Here's the drawing with two shaded views (mm, measured from the low corner). I have some questions. A direction names the side the tool comes from. Give positions to 0.01 mm unless a question says otherwise; leave off trailing zeros. Loops run counter-clockwise (first coordinate to the right, second up) from the corner with the lowest first, then second, coordinate; pieces in that order, holes last. Notation, with made-up numbers: (-27, 25.5) - (-16, 25.5) arc R34 ccw to (-16, 61.5) - close; hole circle Ø5 at (-36, -11). An arc over 180 degrees is marked (long way). Use one line per item in the form item = value.
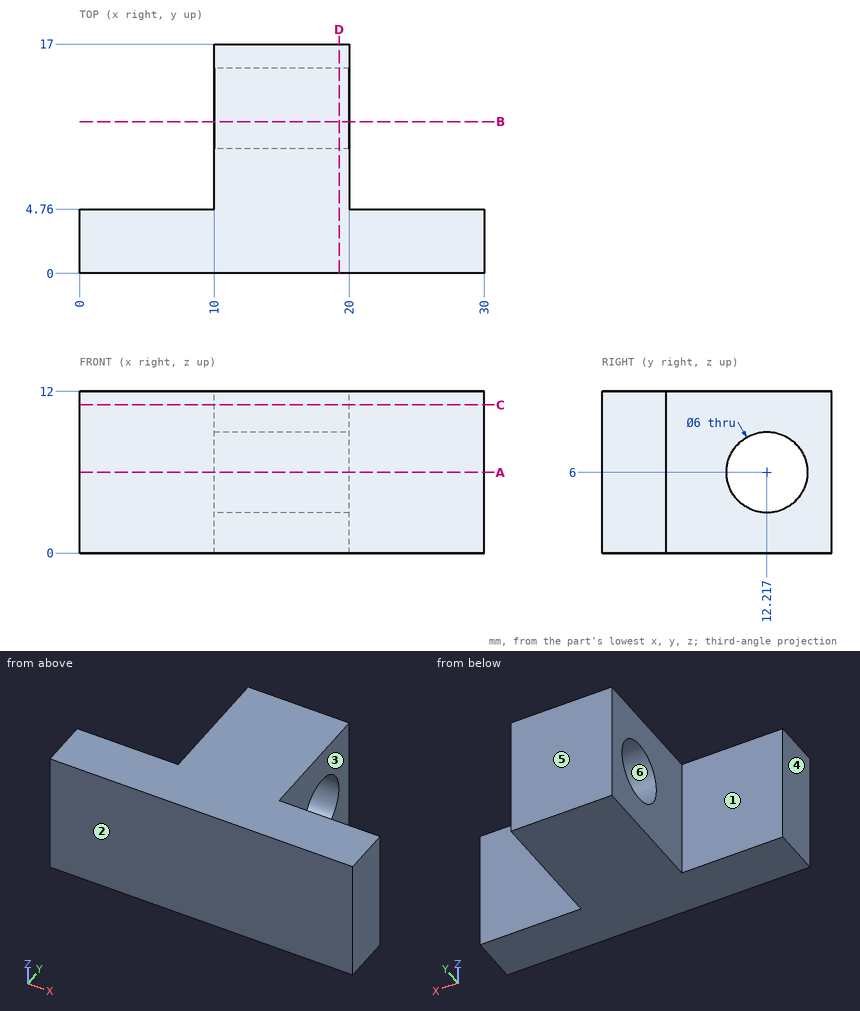
(1) If we section it at C-C (z = 11): List the corners of the cut face in (x, y) for me.
Geometry says:
outline = (0, 0) - (30, 0) - (30, 4.76) - (20, 4.76) - (20, 17) - (10, 17) - (10, 4.76) - (0, 4.76) - close
(2) If we section it at D-D (x = 19.25): List the corners of the cut face in (y, z) for me.
Geometry says:
outline = (0, 0) - (17, 0) - (17, 12) - (0, 12) - close; hole circle Ø6 at (12.22, 6)
(3) If we section it at B-B (y = 11.25): List the corners of the cut face in (x, z) for me, plus the area to 3 significant figures.
Geometry says:
outline = (10, 0) - (20, 0) - (20, 3.16) - (10, 3.16) - close; (10, 8.84) - (20, 8.84) - (20, 12) - (10, 12) - close
area = 63.2 mm²
(4) Thinking about a two-plate mould opening in Y: for the marked faces 4, 5 and 6, which applies, pulls with the +Y half, pulls with the -Y half, needs draft (parallel to the pull), parting line crosses it, or undercut?
Geometry says:
face_4 = needs draft
face_5 = pulls with the +Y half
face_6 = undercut
(5) For P1, Ø3.5, axis at y = 10, z = 3.5, coming from the -X side; P2, Ø5, axis at x = 25.5, z = 8, coming from the +Y side, each with a flat end and sliding along its axis, tell me the tip position at first contact or that it passes through.
Geometry says:
P1 = 10
P2 = 4.76
(6) If I drill on probe 1 along Y at (x, z) = (14.5, 6); probe 2 along Y at (x, z) = (9.75, 3.25); probe 3 along X at (y, z) = (16, 8.5), over which ranges is the centre line in solid material (lowest first)?
Geometry says:
probe_1 = 0 to 9.22, 15.22 to 17
probe_2 = 0 to 4.76
probe_3 = 10 to 20
(7) For the marked faces 1, 2 and 3, which set-ups out of +Z, -Z, +X, -X, +Y, -Y let a thin tool reach every point of the face, with its end or its side?
Geometry says:
face_1 = +Z, -Z, -X, +Y
face_2 = +Z, -Z, +X, -X, -Y
face_3 = +Z, -Z, +X, +Y
(8) If we section it at A-A (z = 6): List the corners of the cut face in (x, y) for me.
Geometry says:
outline = (0, 0) - (30, 0) - (30, 4.76) - (20, 4.76) - (20, 9.22) - (10, 9.22) - (10, 4.76) - (0, 4.76) - close; (10, 15.22) - (20, 15.22) - (20, 17) - (10, 17) - close
